from build123d import *

# Parameters (mm, degrees)
F0_R     = 2.5
F0_R_2   = 2
F1_DEPTH = 2


with BuildPart() as f1:
    # F0 (on Top) → F1 (new body)
    with BuildSketch(Plane.XY):
        with BuildLine():
            Line((28.394605, 56.648372), (-35.605395, 56.648372))
            ThreePointArc((-35.605395, 56.648372), (-42.676463, 53.71944), (-45.605395, 46.648372))
            Line((-45.605395, 46.648372), (-45.605395, -19.851628))
            ThreePointArc((-45.605395, -19.851628), (-42.676463, -26.922696), (-35.605395, -29.851628))
            Line((-35.605395, -29.851628), (28.394605, -29.851628))
            ThreePointArc((28.394605, -29.851628), (35.465673, -26.922696), (38.394605, -19.851628))
            Line((38.394605, -19.851628), (38.394605, 46.648372))
            ThreePointArc((38.394605, 46.648372), (35.465673, 53.71944), (28.394605, 56.648372))
        make_face()
        with Locations((-35.605395, -19.851628)):
            Circle(F0_R, mode=Mode.SUBTRACT)
        with Locations((-36.105395, -7.851628)):
            Circle(F0_R_2, mode=Mode.SUBTRACT)
        with Locations((28.894605, -7.851628)):
            Circle(F0_R_2, mode=Mode.SUBTRACT)
        with Locations((-35.605395, 46.648372)):
            Circle(F0_R, mode=Mode.SUBTRACT)
        with BuildLine():
            Line((16.394605, -19.851628), (16.394605, 46.648372))
            ThreePointArc((16.394605, 46.648372), (19.394605, 49.648372), (22.394605, 46.648372))
            Line((22.394605, 46.648372), (22.394605, -19.851628))
            ThreePointArc((22.394605, -19.851628), (19.394605, -22.851628), (16.394605, -19.851628))
        make_face(mode=Mode.SUBTRACT)
        with BuildLine():
            Line((34.856625, 21.471174), (31.856625, 4.457329))
            ThreePointArc((31.856625, 4.457329), (28.960485, 2.42943), (26.932586, 5.32557))
            Line((26.932586, 5.32557), (29.932586, 22.339415))
            ThreePointArc((29.932586, 22.339415), (32.828726, 24.367314), (34.856625, 21.471174))
        make_face(mode=Mode.SUBTRACT)
    extrude(amount=F1_DEPTH)


solid = f1.part
Input: part model. Units: mm. Frame: model coordinates. A direction names the side the tool comes from. Coordinates: 2 decimals unless noted, no trailing zeros. Write each loop counter-clockwise with the first axis right and the second up, starting at its lowest first coordinate (ties: lowest second). Pieces come first, ordered by that corner, then holes. Notation, with made-up numbers: M 79,82.5 L 129,82.5 A8 cw 129,97.5 Z; hole C 68,-23.75 d2. An arc over 180 degrees is marked long. Answer as a JSON object with one key per item and string values. Group by question number.
(1) Section B-B on z = 0.7. Output: boundary loops of the cut face in (x, y).
(2) Mould query, pull axis Y, two halves, no side actions, for faces 3 (the face through (35.39, -27, 0.99)), 4 (the face through (-38.103, -7.764, 0.986)), 5 (the face through (35.543, 53.641, 0.986)). Classes: pulls with the +Y half, pulls with the -Y half, needs draft (parallel to the pull), parting line crosses it, or undercut.
(3) Ray query, line 1 along X through (y, z) = (-1.5, 0.35); line 2 along X through (y, z) = (-21.5, 1.3); line 3 along Y through (x, z) = (-35.5, 0.6). Return the intervals inside material, ascending. Write a range as [from, to].
(4) Section D-D on y = 18.5. Output: boundary loops of the cut face in (x, z), plus the area to 3 significant figures.
(5) Section A-A on y = 27.5. Output: boundary loops of the cut face in (x, z), plus the area to 3 significant figures.
(6) Section C-C on x = 19. Output: boundary loops of the cut face in (y, z), plus the area to 3 significant figures.
(7) Set-up query: faces 1 (the face through (28.41, 13.71, 0.99)), 2 (the face through (-45.605, 14, 1)). Return all of +Z, -Z, +X, -X, +Y, -Y with unobstructed straight access to the full face (end or side cutting, diameter ignored); none if empty.
Result set:
{
 "1": {"outline": "M -45.61,-19.85 A10 ccw -35.61,-29.85 L 28.39,-29.85 A10 ccw 38.39,-19.85 L 38.39,46.65 A10 ccw 28.39,56.65 L -35.61,56.65 A10 ccw -45.61,46.65 Z; hole C -35.61,-19.85 d5; hole C -36.11,-7.85 d4; hole C -35.61,46.65 d5; hole M 16.39,-19.85 A3 ccw 22.39,-19.85 L 22.39,46.65 A3 ccw 16.39,46.65 Z; hole C 28.89,-7.85 d4; hole M 26.93,5.33 A2.5 ccw 31.86,4.46 L 34.86,21.47 A2.5 ccw 29.93,22.34 Z"},
 "2": {"face 3": "pulls with the -Y half", "face 4": "undercut", "face 5": "pulls with the +Y half"},
 "3": {"line 1": "x = [-45.61, 16.39], [22.39, 38.39]", "line 2": "x = [-45.47, -37.48], [-33.73, 16.89], [21.9, 38.26]", "line 3": "y = [-29.85, -22.35], [-17.35, -9.76], [-5.95, 44.15], [49.15, 56.65]"},
 "4": {"outline": "M -45.61,0 L 16.39,0 L 16.39,2 L -45.61,2 Z; M 22.39,0 L 29.26,0 L 29.26,2 L 22.39,2 Z; M 34.33,0 L 38.39,0 L 38.39,2 L 34.33,2 Z", "area": "146 mm2"},
 "5": {"outline": "M -45.61,0 L 16.39,0 L 16.39,2 L -45.61,2 Z; M 22.39,0 L 38.39,0 L 38.39,2 L 22.39,2 Z", "area": "156 mm2"},
 "6": {"outline": "M -29.85,0 L -22.83,0 L -22.83,2 L -29.85,2 Z; M 49.62,0 L 56.65,0 L 56.65,2 L 49.62,2 Z", "area": "28.1 mm2"},
 "7": {"face 1": "+Z, -Z", "face 2": "+Z, -Z, -X, +Y, -Y"}
}
